Build history of the part. All positions in model axes, mm. Coordinates: 2 decimals unless noted, no trailing zeros. Loops run counter-clockwise (first coordinate to the right, second up) from the corner with the lowest first, then second, coordinate; pieces in that order, holes last.
(1) Slice it at A-A (z = 1900). Give the cut face in (x, y).
(2) Wall check: L1, parallel to Y at x = -21, z = 1900; L2, parallel to Z at x = -44, y = 71; L3, parallel to Z at x = -53, y = 74.5. Give the ranges that are in metal, low to high.
(3) Flat gauge pins, fed straight in: P1, Ø24, axis at y = 86.65, z = 1900, coming from the +X side; P2, Ø2, axis at x = -49, y = 110, coming from the -Z side. Where does each tip first touch, or does it go through?
from build123d import *

# Parameters (mm, degrees)
F1_DEPTH = 2100
F3_D     = 40


with BuildPart() as f1:
    # F0 (on Top) → F1 (new body)
    with BuildSketch(Plane.XY):
        Polygon((-34.255523, 181.653569), (-65, 181.653569), (-65, -8.346431), (65, -8.346431), (65, 181.653569), (34.255523, 181.653569), align=None)
    extrude(amount=F1_DEPTH)

    # F3 (through all)
    with Locations(Plane.YZ.offset(65)):
        with Locations((86.653569, 1900)):
            Hole(F3_D / 2)


solid = f1.part
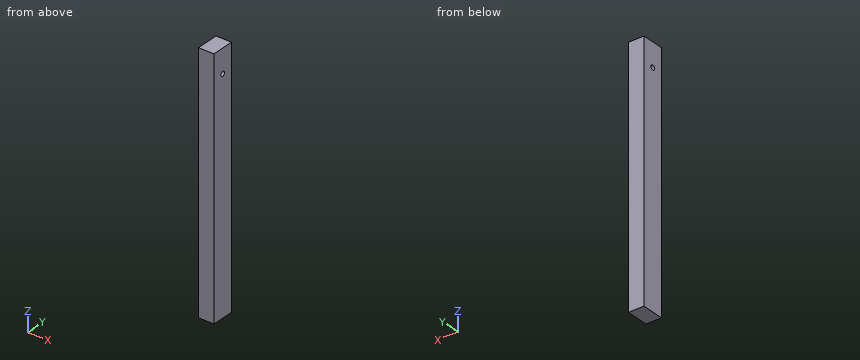
Response values:
1. outline: (-65, -8.35) - (65, -8.35) - (65, 66.65) - (-65, 66.65) - close; (-65, 106.65) - (65, 106.65) - (65, 181.65) - (-65, 181.65) - close
2. L1: y = -8.35 to 66.65, 106.65 to 181.65
2. L2: z = 0 to 1887.55, 1912.45 to 2100
2. L3: z = 0 to 1884.12, 1915.88 to 2100
3. P1: passes through
3. P2: stops at z = 0
